from build123d import *

# Parameters (mm, degrees)
SKETCH1_W           = 40
SKETCH1_H           = 16
BOSS_EXTRUDE1_DEPTH = 26
SKETCH6_R           = 6
CUT_EXTRUDE1_DEPTH  = 61


with BuildPart() as part:
    # Sketch1 → Boss-Extrude1 (new body)
    with BuildSketch(Plane.XY):
        with BuildLine():
            Line((2, 0), (58, 0))
            ThreePointArc((58, 0), (59.414213562, 0.585786438), (60, 2))
            Line((60, 2), (60, 24))
            ThreePointArc((60, 24), (59.414213562, 25.414213562), (58, 26))
            Line((58, 26), (2, 26))
            ThreePointArc((2, 26), (0.585786438, 25.414213562), (0, 24))
            Line((0, 24), (0, 2))
            ThreePointArc((0, 2), (0.585786438, 0.585786438), (2, 0))
        make_face()
        with Locations((30, 13)):
            Rectangle(SKETCH1_W, SKETCH1_H, mode=Mode.SUBTRACT)
    extrude(amount=BOSS_EXTRUDE1_DEPTH)

    # Sketch6 → Cut-Extrude1 (cut, through all)
    with BuildSketch(Plane(origin=(60, 0, 0), x_dir=(0, 0, -1), z_dir=(1, 0, 0))):
        with Locations((-13, 13)):
            Circle(SKETCH6_R)
    extrude(amount=-CUT_EXTRUDE1_DEPTH, mode=Mode.SUBTRACT)


solid = part.part
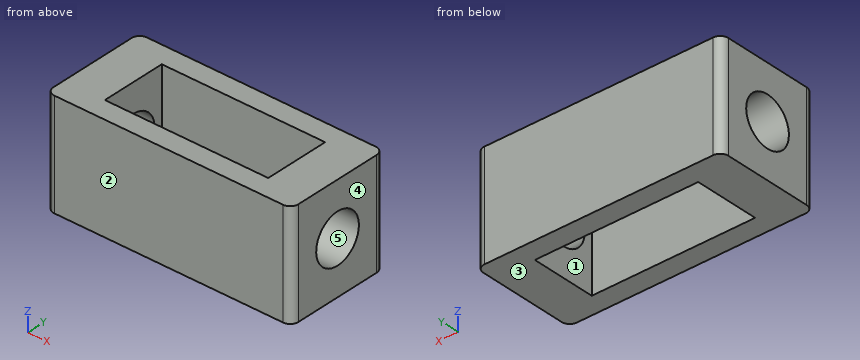
For this review, take the finished solid that the model builds, in its own axes (mm). Face numbers are marked on the shaded views. A direction names the side the tool comes from. Give positions to 0.01 mm unless a question says otherwise; leave off trailing zeros. Order: outer loops, then holes, each group sorted by start corner. A loop starts at its lowest first (then second) coordinate and runs counter-clockwise, first axis right, second up. Notation, with made-up numbers: M -38.5,72 L -18.5,72 A19 ccw -18.5,104 Z; hole C 62.5,4 d6. An arc over 180 degrees is marked long. Answer in a Markdown table with one row per item. Add a question column.
(1) Consider section A-A on y = 20. State the section outline as (x, z) points.
(2) For the marked faces 1 and 2, list the 3-axis set-ups (+Z, -Z, +X, -X, +Y, -Y) from which the entire face can be reached by the end or side of a thin tool; tool diameter is ignored.
(3) Mouldability with a two-part tool opening along Z and no side actions: class the marked faces 3, 4 and 5 as +Z half, -Z half, draft (parallel to the pull), parting line (faces both ways), or undercut.
(4) Wall thickness on probe 1 along Y at (x, z) = (53.5, 13); probe 2 along X at (y, z) = (8.25, 4.75); probe 3 along Y at (x, z) = (25.5, 7.5): over which ranges is each line inside the solid? List them lowest first. Write a range as [from, to].
(5) Consider section D-D on z = 13. State the section outline as (x, y) points, and give its area (3 significant figures).
(6) Consider section C-C on x = 25.5. State the section outline as (y, z) points, and give its area (3 significant figures).
(7) For pin 1 (1 mm diameter, centred on x = 33, z = 12.5, fed in from -Y), flat-tipped, find the tip position at first contact; note if it passes through.
(8) Consider section B-B on y = 13. State the section outline as (x, z) points.
Evaluation:
| question | item | result |
|---|---|---|
| 1 | outline | M 0,0 L 10,0 L 10,26 L 0,26 Z; M 50,0 L 60,0 L 60,26 L 50,26 Z |
| 2 | face 1 | +Z, -Z |
| 2 | face 2 | +Z, -Z, +X, -X, -Y |
| 3 | face 3 | -Z half |
| 3 | face 4 | draft |
| 3 | face 5 | undercut |
| 4 | probe 1 | y = [0, 7], [19, 26] |
| 4 | probe 2 | x = [0, 10], [50, 60] |
| 4 | probe 3 | y = [0, 5], [21, 26] |
| 5 | outline | M 0,2 A2 ccw 2,0 L 58,0 A2 ccw 60,2 L 60,7 L 50,7 L 50,5 L 10,5 L 10,7 L 0,7 Z; M 0,19 L 10,19 L 10,21 L 50,21 L 50,19 L 60,19 L 60,24 A2 ccw 58,26 L 2,26 A2 ccw 0,24 Z |
| 5 | area | 677 mm^2 |
| 6 | outline | M 0,0 L 5,0 L 5,26 L 0,26 Z; M 21,0 L 26,0 L 26,26 L 21,26 Z |
| 6 | area | 260 mm^2 |
| 7 | pin 1 | stops at y = 0 |
| 8 | outline | M 0,0 L 10,0 L 10,7 L 0,7 Z; M 0,19 L 10,19 L 10,26 L 0,26 Z; M 50,0 L 60,0 L 60,7 L 50,7 Z; M 50,19 L 60,19 L 60,26 L 50,26 Z |
